Read the model definition and answer for the solid it produces. Units are mm, in the model's axes. A direction names the side the tool comes from. Give positions to 0.01 mm unless a question says otherwise; leave off trailing zeros. Write each loop counter-clockwise with the first axis right and the second up, starting at its lowest first coordinate (ties: lowest second). Pieces come first, ordered by that corner, then holes. Notation, with made-up numbers: (-31, 21.25) -> (15, 21.25) arc R19 cw to (15, 55.25) -> close; hole circle Ø5 at (-10, 31). An arc over 180 degrees is marked (long way). Write item = value, one per line.
from build123d import *

# Parameters (mm, degrees)
SKETCH1_W                    = 209.476
SKETCH1_H                    = 175.514
BASE_FLANGE1_DEPTH           = 2.3622
EDGE_FLANGE4_STRIP_W         = 14.1688
EDGE_FLANGE4_STRIP_H         = 2.3622
EDGE_FLANGE4_STRIP_CUT_DEPTH = 209.476
EDGE_FLANGE4_DEPTH           = 209.476
CUT_EXTRUDE1_DEPTH           = 152.058528265
SKETCH38_R                   = 2.413
CUT_EXTRUDE2_DEPTH           = 152.058528265
SKETCH39_R                   = 2.413
CUT_EXTRUDE3_DEPTH           = 152.058528265


# Sheet-metal steps are written as plain solids
with BuildPart() as part:
    # Sketch1 → Base-Flange1 (new body)
    with BuildSketch(Plane(origin=(0, 0, 0), x_dir=(1, 0, 0), z_dir=(0, 1, 0))):
        with Locations((15.34, 0)):
            Rectangle(SKETCH1_W, SKETCH1_H)
    extrude(amount=-BASE_FLANGE1_DEPTH)

    # Edge-Flange4 strip (across the edge) → Edge-Flange4 strip cut (cut)
    with BuildSketch(Plane(origin=(120.078, -2.3622, 87.757), x_dir=(0, 0, -1), z_dir=(-1, 0, 0))):
        with Locations((-4.7244, -1.1811)):
            Rectangle(EDGE_FLANGE4_STRIP_W, EDGE_FLANGE4_STRIP_H)
    extrude(amount=EDGE_FLANGE4_STRIP_CUT_DEPTH, mode=Mode.SUBTRACT)

    # Edge-Flange4 section (across the edge) → Edge-Flange4 (add)
    with BuildSketch(Plane(origin=(120.078, -2.3622, 87.757), x_dir=(0, 0, -1), z_dir=(-1, 0, 0))):
        with BuildLine():
            Line((-2.3622, 2.36), (-2.3622, 16.6878))
            Line((-2.3622, 16.6878), (0, 16.6878))
            Line((0, 16.6878), (0, 2.36))
            ThreePointArc((0, 2.36), (0.691227996, 0.691227996), (2.36, 0))
            Line((2.36, 0), (2.36, -2.3622))
            ThreePointArc((2.36, -2.3622), (-0.979099642, -0.979099642), (-2.3622, 2.36))
        make_face()
    extrude(amount=EDGE_FLANGE4_DEPTH)

    # Sketch36 → Cut-Extrude1 (cut, through all)
    with BuildSketch(Plane.XZ.offset(2.3622)):
        Polygon((-94.1202, 26.6192), (58.938, -68.707), (140.022587244, -68.707), (140.022587244, -102.574234495), (-121.93122604, -102.574234495), (-121.93122604, 26.6192), align=None)
    extrude(amount=-CUT_EXTRUDE1_DEPTH, mode=Mode.SUBTRACT)

    # Sketch38 → Cut-Extrude2 (cut, through all)
    with BuildSketch(Plane.XZ.offset(2.3622)):
        with Locations(Location((-82.2341, 73.967, 0), (0, 0, 270))):
            Circle(SKETCH38_R)
        with Locations(Location((-82.2341, 62.537, 0), (0, 0, 270))):
            Circle(SKETCH38_R)
        with Locations(Location((-82.2341, 51.107, 0), (0, 0, 270))):
            Circle(SKETCH38_R)
        with Locations(Location((-82.2341, 39.677, 0), (0, 0, 270))):
            Circle(SKETCH38_R)
    extrude(amount=-CUT_EXTRUDE2_DEPTH, mode=Mode.SUBTRACT)

    # Sketch39 → Cut-Extrude3 (cut, through all)
    with BuildSketch(Plane.XZ.offset(2.3622)):
        with Locations(Location((112.9141, 73.967, 0), (0, 0, 270))):
            Circle(SKETCH39_R)
        with Locations(Location((112.9141, 59.168910638, 0), (0, 0, 270))):
            Circle(SKETCH39_R)
        with Locations(Location((112.9141, 44.370821275, 0), (0, 0, 270))):
            Circle(SKETCH39_R)
        with Locations(Location((112.9141, 29.572731913, 0), (0, 0, 270))):
            Circle(SKETCH39_R)
        with Locations(Location((112.9141, 14.774642551, 0), (0, 0, 270))):
            Circle(SKETCH39_R)
        with Locations(Location((112.9141, -0.023446812, 0), (0, 0, 270))):
            Circle(SKETCH39_R)
        with Locations(Location((112.9141, -14.821536174, 0), (0, 0, 270))):
            Circle(SKETCH39_R)
        with Locations(Location((112.9141, -29.619625536, 0), (0, 0, 270))):
            Circle(SKETCH39_R)
        with Locations(Location((112.9141, -44.417714899, 0), (0, 0, 270))):
            Circle(SKETCH39_R)
    extrude(amount=-CUT_EXTRUDE3_DEPTH, mode=Mode.SUBTRACT)


solid = part.part
(1) The part is cut by section B-B on z = -51. Determine the outline of the cut face in (x, y), plus the area to 3 significant figures.
Checks:
outline = (30.51, -2.36) -> (120.08, -2.36) -> (120.08, 0) -> (30.51, 0) -> close
area = 212 mm²
(2) The part is cut by section A-A on x = 102. Determine the outline of the cut face in (y, z), plus the area to 3 significant figures.
Checks:
outline = (-19.05, 87.76) -> (-4.72, 87.76) arc R2.36 cw to (-2.36, 85.4) -> (-2.36, -68.71) -> (0, -68.71) -> (0, 85.4) arc R4.72 ccw to (-4.72, 90.12) -> (-19.05, 90.12) -> close
area = 411 mm²
(3) Consider L1, parallel to Y at x = 76.5, z = 56; L2, parallel to Z at x = 110.5, y = -9; L3, parallel to X at y = -2, z = 16.5. Determine where each line is inside the solid, lowest interval first.
Checks:
L1 = -2.36 to 0
L2 = 87.76 to 90.12
L3 = -77.87 to 111.23, 114.6 to 120.08
(4) Given P1, Ø6.5, axis at x = 112.91, z = 59.17, coming from the -Y side; P2, Ø5, axis at x = 90, y = -12, coming from the -Z side; P3, Ø10, axis at x = -45.5, y = -3, coming from the -Z side, each flat-ended and moving along its own axis, determine where each tip first touches the part or whether it passes through.
Checks:
P1 = -2.36
P2 = 87.76
P3 = -6.75
(5) A tool of negligible diameter and unlimited length cuts with its end or side. For faces 1 (the flat face through (37, -2.362, 24)), 2 (the cylindrical face through (-83.702, -1.198, 64.452)), from which of +Z, -Z, +X, -X, +Y, -Y can it reach the whole face along a straight path? Write none if from no direction.
Checks:
face_1 = -Z, +X, -X, -Y
face_2 = +Y, -Y
(6) The part is cut by section C-C on x = -42. Determine the outline of the cut face in (y, z), plus the area to 3 significant figures.
Checks:
outline = (-19.05, 87.76) -> (-4.72, 87.76) arc R2.36 cw to (-2.36, 85.4) -> (-2.36, -5.84) -> (0, -5.84) -> (0, 85.4) arc R4.72 ccw to (-4.72, 90.12) -> (-19.05, 90.12) -> close
area = 263 mm²
(7) For a pull along X with two mould halves and no side action, classify faces 3 (the flat face through (37, 0, 24)), 4 (the cylindrical face through (111.446, -1.198, 61.084)), 5 (the flat face through (120.078, -1, 10)) as released by +X, released by -X, zero draft, split by the parting line, or undercut.
Checks:
face_3 = zero draft
face_4 = undercut
face_5 = released by +X
